Check sheet for the drawn part. Datum: minimum x, y, z corner. Units: mm. A direction names the side the tool comes from. Round coordinates to 2 decimals unless told otherwise and drop trailing zeros. Write each loop counter-clockwise with the first axis right and the second up, starting at its lowest first coordinate (ties: lowest second). Pieces come first, ordered by that corner, then holes. Notation, with made-up numbers: M -27.5,-15.5 L -8.5,-15.5 A17 ccw -8.5,-7.5 Z; hole C -18,-4.75 d4. An arc over 180 degrees is marked long. Put each result on its own line as item: value.
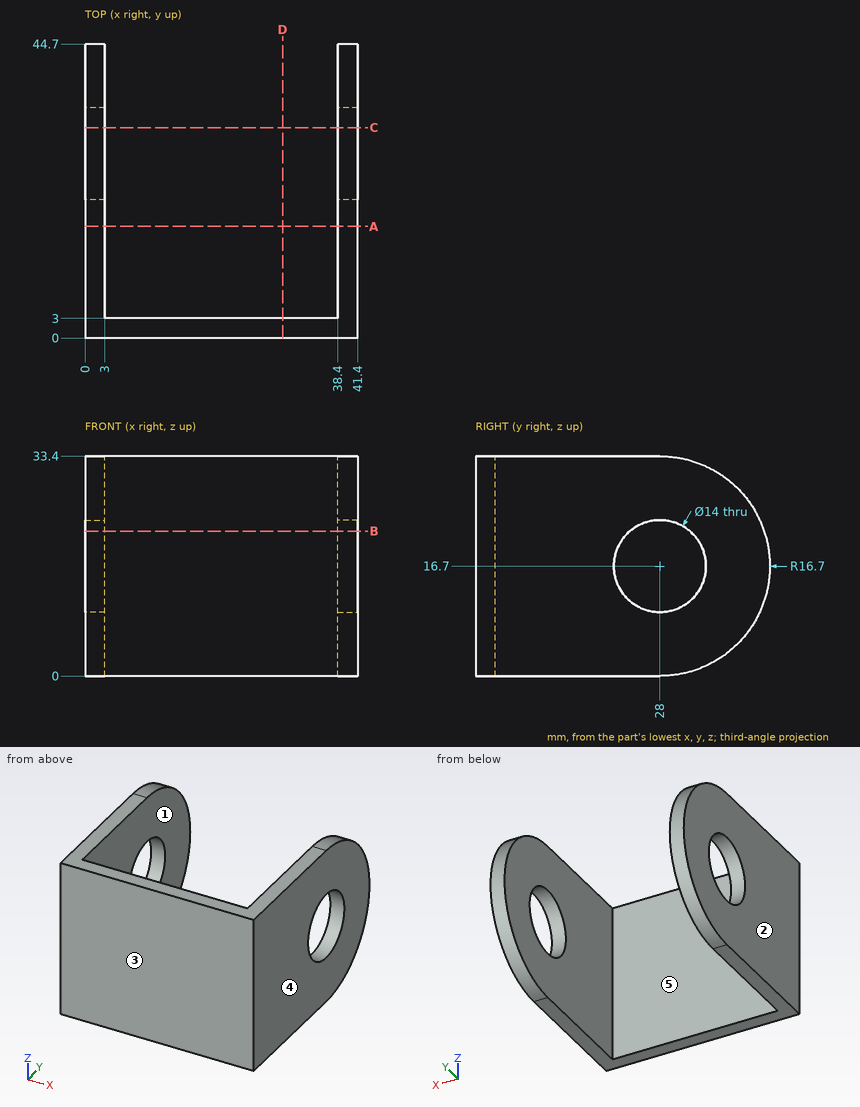
1. Cross-section at D-D (x = 30). Enter the section's corners in (y, z).
Computed values:
outline: M 0,0 L 3,0 L 3,33.4 L 0,33.4 Z
2. Scan lines: probe 1 along Y at (x, z) = (39.55, 16.7); probe 2 along X at (y, z) = (13.5, 30); probe 3 along Y at (x, z) = (13, 24.5). Record each from-to range of solid material in increasing order.
Computed values:
probe 1: y = 0 to 21, 35 to 44.7
probe 2: x = 0 to 3, 38.4 to 41.4
probe 3: y = 0 to 3
3. Access from +Z, -Z, +X, -X, +Y, -Y to the whole of each face (thin tool, end or side, straight path). Record for the marked faces 1 and 2.
Computed values:
face 1: +Z, -Z, +Y
face 2: +Z, -Z, -X, +Y, -Y
4. Depth check by flat-ended pin: pin 1 Ø4 at (x, y) = (4.5, 35) entering from +Z; pin 2 Ø5 at (y, z) = (34, 10.5) entering from -X; pin 3 Ø12.5 at (y, z) = (28, 16.7) entering from +X; pin 4 Ø10 at (x, z) = (26, 24) entering from +Y. Enter the tip coordinate at first touch or a pass-through.
Computed values:
pin 1: stops at z = 32.41
pin 2: stops at x = 0
pin 3: passes through
pin 4: stops at y = 3
5. Release check for a two-part mould opening along X. For the marked faces 3, 4 and 5 record: +X half, -X half, draft (parallel to the pull), parting line (faces both ways), or undercut.
Computed values:
face 3: draft
face 4: +X half
face 5: undercut
6. Cross-section at A-A (y = 17). Enter the section's corners in (x, z).
Computed values:
outline: M 0,0 L 3,0 L 3,33.4 L 0,33.4 Z; M 38.4,0 L 41.4,0 L 41.4,33.4 L 38.4,33.4 Z
7. Cross-section at C-C (y = 32). Enter the section's corners in (x, z), then the cut area to 3 significant figures.
Computed values:
outline: M 0,0.49 L 3,0.49 L 3,10.96 L 0,10.96 Z; M 0,22.44 L 3,22.44 L 3,32.91 L 0,32.91 Z; M 38.4,0.49 L 41.4,0.49 L 41.4,10.96 L 38.4,10.96 Z; M 38.4,22.44 L 41.4,22.44 L 41.4,32.91 L 38.4,32.91 Z
area: 126 mm2
8. Cross-section at B-B (z = 22). Enter the section's corners in (x, y).
Computed values:
outline: M 0,0 L 41.4,0 L 41.4,23.43 L 38.4,23.43 L 38.4,3 L 3,3 L 3,23.43 L 0,23.43 Z; M 0,32.57 L 3,32.57 L 3,43.84 L 0,43.84 Z; M 38.4,32.57 L 41.4,32.57 L 41.4,43.84 L 38.4,43.84 Z
